Part print with two shaded views. Sizes in mm from the minimum x, y, z corner. A direction names the side the tool comes from. Give positions to 0.01 mm unless a question says otherwise; leave off trailing zeros. Loops run counter-clockwise (first coordinate to the right, second up) from the corner with the lowest first, then second, coordinate; pieces in that order, holes last. Notation, with made-up numbers: M 19.5,2 L 34.5,2 A29 ccw 34.5,41 Z; hole C -33,80.5 d10. An arc over 180 degrees is marked long. Answer as a JSON object with one key per item and string values. Group by question number.
1. Slice it at C-C (y = 2.9). List the corners of the cut face in (x, z), then the cut area to 3 significant figures.
2. Drop flat-ended pins along their axis: pin 1 Ø4 at (x, z) = (6, 2) entering from -Y; pin 2 Ø2 at (y, z) = (3, 9) entering from -X; pin 3 Ø1.5 at (x, y) = (1.5, 3) entering from -Z. Give the stop position or say it passes through.
3. Mould opens along Z. For the marked faces 3, 4, 5 and 6 say: released by +Z, released by -Z, zero draft, split by the parting line, or undercut.
4. 3-axis set-ups, long thin cutter, end or side, ignore diameter. For the marked faces 1 and 2: which of +Z, -Z, +X, -X, +Y, -Y reach the whole face in a straight line?
5. Slice it at B-B (x = 8). List the corners of the cut face in (y, z), then the cut area to 3 significant figures.
6. Drill centre lines: line 1 along Z through (x, y) = (7, 4.5); line 2 along Z through (x, y) = (6.25, 0.25); line 3 along X through (y, z) = (4.65, 9.75). Where is each one in solid material? Low to high. Write a range as [from, to].
7. Slice it at A-A (z = 7). List the corners of the cut face in (x, y), then the cut area to 3 significant figures.
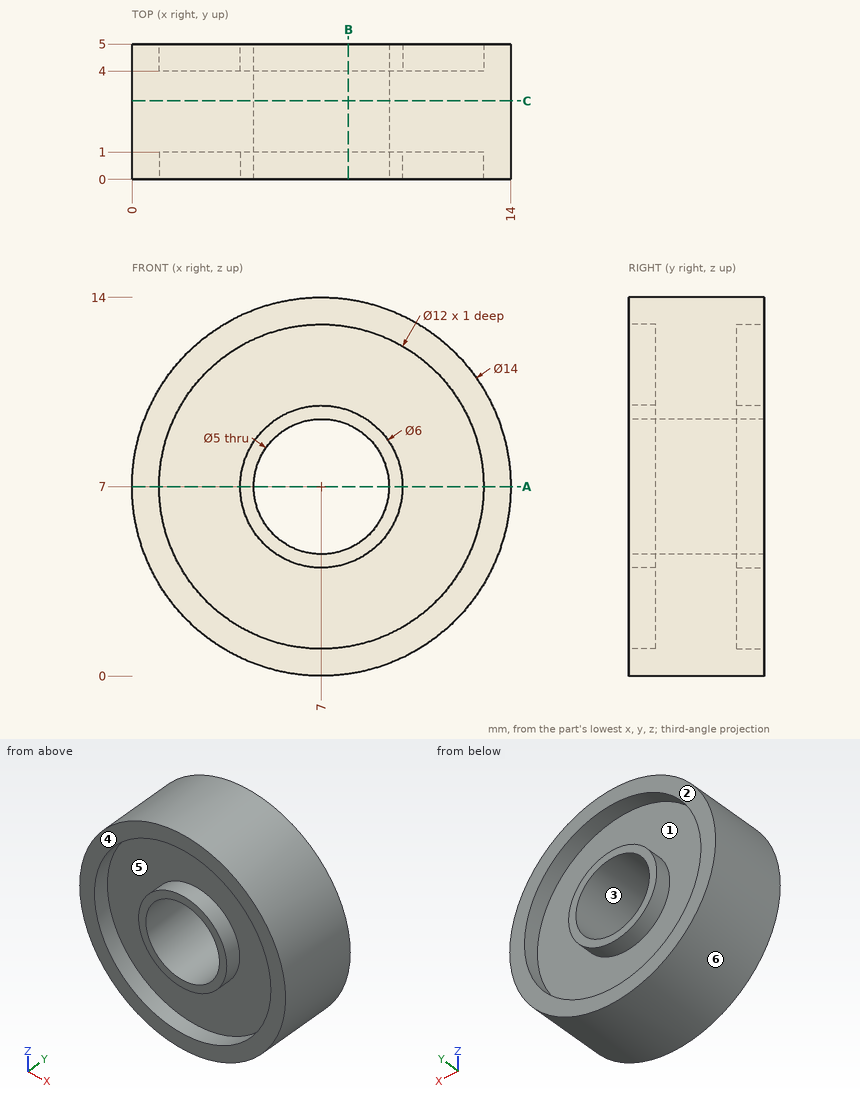
Established:
{
 "1": {"outline": "C 7,7 d14; hole C 7,7 d5", "area": "134 mm^2"},
 "2": {"pin 1": "stops at y = 0", "pin 2": "stops at x = 0.07", "pin 3": "stops at z = 1.86"},
 "3": {"face 3": "undercut", "face 4": "zero draft", "face 5": "undercut", "face 6": "split by the parting line"},
 "4": {"face 1": "+Y", "face 2": "+Z, -Z, +X, -X, +Y"},
 "5": {"outline": "M 0,0.07 L 5,0.07 L 5,1.08 L 4,1.08 L 4,4.17 L 5,4.17 L 5,4.71 L 0,4.71 L 0,4.17 L 1,4.17 L 1,1.08 L 0,1.08 Z; M 0,9.29 L 5,9.29 L 5,9.83 L 4,9.83 L 4,12.92 L 5,12.92 L 5,13.93 L 0,13.93 L 0,12.92 L 1,12.92 L 1,9.83 L 0,9.83 Z", "area": "34.0 mm^2"},
 "6": {"line 1": "z = [0, 1], [4, 4.5], [9.5, 10], [13, 14]", "line 2": "z = [0.04, 1.05], [4.1, 4.62], [9.38, 9.9], [12.95, 13.96]", "line 3": "x = [0.56, 1.67], [5.8, 8.2], [12.33, 13.44]"},
 "7": {"outline": "M 0,0 L 1,0 L 1,1 L 4,1 L 4,0 L 4.5,0 L 4.5,5 L 4,5 L 4,4 L 1,4 L 1,5 L 0,5 Z; M 9.5,0 L 10,0 L 10,1 L 13,1 L 13,0 L 14,0 L 14,5 L 13,5 L 13,4 L 10,4 L 10,5 L 9.5,5 Z", "area": "33.0 mm^2"}
}
